Part model, mm, in its own coordinate system. A direction names the side the tool comes from. Round coordinates to 2 decimals unless told otherwise and drop trailing zeros. Write each loop counter-clockwise with the first axis right and the second up, starting at its lowest first coordinate (ties: lowest second). Pieces come first, ordered by that corner, then holes.
from build123d import *

# Parameters (mm, degrees)
F0_W     = 88.9
F0_H     = 6.350001
F1_DEPTH = 63.5
F2_DEPTH = 222.25


with BuildPart() as f1:
    # F0 (on Top) → F1 (new body)
    with BuildSketch(Plane.XY):
        with Locations((-1.781045, -36.954149)):
            Rectangle(F0_W, F0_H)
    extrude(amount=F1_DEPTH)

    # F0 (on Top) → F2 (join)
    with BuildSketch(Plane.XY):
        Polygon((-46.231045, -33.779149), (-46.231045, 57.660851), (42.668955, 57.660851), (42.668955, -33.779149), (42.668955, -40.12915), (49.018957, -40.12915), (49.018957, 64.010852), (-52.581046, 64.010852), (-52.581046, -40.12915), (-46.231045, -40.12915), align=None)
    extrude(amount=F2_DEPTH)


solid = f1.part
Q1. Two-plate mould, pull along X, no slides. Class faces 1 (the flat face through (-47, 12, 0)), 2 (the flat face through (49.019, 11, 110)), 3 (the flat face through (42.669, 9, 110)): released by +X, released by -X, zero draft, split by the parting line, or undercut.
Q2. Drop flat-ended pins along their axis: P1, Ø1.5, axis at x = 25.5, z = 87.5, coming from the -Y side; P2, Ø5, axis at x = -12, y = -35.5, coming from the +Z side. Give the stop position or say it passes through.
Q3. Saw through at D-D, the plane z = 159. Write the cut outline in (x, y).
Q4. Wall check: line 1 (X direction, y = 35, z = 213); line 2 (Y direction, x = -46, z = 51); line 3 (Y direction, x = -1, z = 150.5). Give the ranges that are in metal, low to high.
Q5. Saw through at B-B, the plane x = 22. Write the cut outline in (y, z).
Q6. Saw through at A-A, the plane y = 23.5. Write the cut outline in (x, z), and give its area (3 significant figures).
Q7. Tool access for faces 4 (the flat face through (46, -40.129, 110)), 5 (the flat face through (-2, -33.779, 31)), 6 (the flat face through (-2, -37, 63.5)): list every direction of +Z, -Z, +X, -X, +Y, -Y with a clear straight run to the whole face (end or side of a thin tool).
Q8. Saw through at C-C, the plane z = 26. Write the cut outline in (x, y).
Computed:
1. face 1: zero draft
1. face 2: released by +X
1. face 3: undercut
2. P1: stops at y = 57.66
2. P2: stops at z = 63.5
3. outline: (-52.58, -40.13) - (-46.23, -40.13) - (-46.23, 57.66) - (42.67, 57.66) - (42.67, -40.13) - (49.02, -40.13) - (49.02, 64.01) - (-52.58, 64.01) - close
4. line 1: x = -52.58 to -46.23, 42.67 to 49.02
4. line 2: y = -40.13 to -33.78, 57.66 to 64.01
4. line 3: y = 57.66 to 64.01
5. outline: (-40.13, 0) - (-33.78, 0) - (-33.78, 63.5) - (-40.13, 63.5) - close; (57.66, 0) - (64.01, 0) - (64.01, 222.25) - (57.66, 222.25) - close
6. outline: (-52.58, 0) - (-46.23, 0) - (-46.23, 222.25) - (-52.58, 222.25) - close; (42.67, 0) - (49.02, 0) - (49.02, 222.25) - (42.67, 222.25) - close
6. area: 2,820 mm2
7. face 4: +Z, -Z, +X, -X, -Y
7. face 5: +Z, -Z
7. face 6: +Z, -Y
8. outline: (-52.58, -40.13) - (49.02, -40.13) - (49.02, 64.01) - (-52.58, 64.01) - close; hole (-46.23, -33.78) - (42.67, -33.78) - (42.67, 57.66) - (-46.23, 57.66) - close
